Verification items for the finished model (mm, model axes). A direction names the side the tool comes from. Give positions to 0.01 mm unless a question says otherwise; leave off trailing zeros. Loops run counter-clockwise (first coordinate to the right, second up) from the corner with the lowest first, then second, coordinate; pieces in that order, holes last. Notation, with made-up numbers: (30, -17.75) -> (81, -17.75) arc R31 cw to (81, 6.25) -> close; hole circle Ø5 at (19, 3). An arc over 180 degrees is marked (long way). Answer in a Markdown table with one row per item. Add a question column.
Q1. Section check A-A on z = 7.5. Enter the section's corners in (x, y), and give its area (3 significant figures).
Q2. Section check B-B on x = -133. Enter the section's corners in (y, z), and give its area (3 significant figures).
Q3. Gauge pin test, flat ends, axial feed: P1, Ø1.5, axis at y = -55.5, z = 8.5, coming from the +X side; P2, Ø3, axis at x = 122.5, z = 5, coming from the -Y side; P3, Ø3, axis at y = -41.5, z = 1.5, coming from the +X side. Record the tip position at first contact, or that the pin passes through.
Q4. Section check C-C on y = -69. Enter the section's corners in (x, z).
Q5. Set-up check for faces 5 (the face through (-16.557, 26.311, 4.93)), 6 (the face through (120, -25, 5)), 7 (the face through (1, 4, 0)): record each of +Z, -Z, +X, -X, +Y, -Y from which the full face is reachable in a straight line by a thin tool's end or side.
Q6. Material ranges on probe 1 along X at (y, z) = (19, 2); probe 2 along X at (y, z) = (15.5, 5.5); probe 3 along X at (y, z) = (37.5, 3.25), recorded low to high.
Q7. Release check for a two-part mould opening along X. For faces 1 (the face through (142, 50, 5)), 2 (the face through (16.517, 26.689, 4.93)), 3 (the face through (-145.83, -7.04, 4.93)), 4 (the face through (0, 30, 5)) record: pulls with the +X half, pulls with the -X half, needs draft (parallel to the pull), parting line crosses it, or undercut.
```python
from build123d import *

# Parameters (mm, degrees)
BOSS_EXTRUDE1_DEPTH = 10


with BuildPart() as part:
    # Sketch1 → Boss-Extrude1 (new body)
    with BuildSketch(Plane.XY):
        with BuildLine():
            Line((67, 50), (220, 50))
            Line((220, 50), (158.952536164, 7.254105633))
            ThreePointArc((158.952536164, 7.254105633), (145.965681261, -6.810123789), (140, -25))
            Line((140, -25), (99.563224144, -25))
            ThreePointArc((99.563224144, -25), (32.234251016, -51.062124878), (0, -115.663812449))
            ThreePointArc((0, -115.663812449), (-32.234251016, -51.062124878), (-99.563224144, -25))
            Line((-99.563224144, -25), (-140, -25))
            ThreePointArc((-140, -25), (-145.965681261, -6.810123789), (-158.952536164, 7.254105633))
            Line((-158.952536164, 7.254105633), (-220, 50))
            Line((-220, 50), (-67, 50))
            ThreePointArc((-67, 50), (-51.137889855, 20.020793424), (-17.95554779, 13))
            Line((-17.95554779, 13), (-15.117733438, 40))
            Line((-15.117733438, 40), (-12, 27.49545417))
            ThreePointArc((-12, 27.49545417), (0, 30), (12, 27.49545417))
            Line((12, 27.49545417), (15.117733438, 40))
            Line((15.117733438, 40), (17.95554779, 13))
            ThreePointArc((17.95554779, 13), (51.137889855, 20.020793424), (67, 50))
        make_face()
    extrude(amount=BOSS_EXTRUDE1_DEPTH)


solid = part.part
```
Taken from the geometry:
| question | item | result |
|---|---|---|
| 1 | outline | (-220, 50) -> (-158.95, 7.25) arc R45 cw to (-140, -25) -> (-99.56, -25) arc R100 cw to (0, -115.66) arc R100 cw to (99.56, -25) -> (140, -25) arc R45 cw to (158.95, 7.25) -> (220, 50) -> (67, 50) arc R40 cw to (17.96, 13) -> (15.12, 40) -> (12, 27.5) arc R30 ccw to (-12, 27.5) -> (-15.12, 40) -> (-17.96, 13) arc R40 cw to (-67, 50) -> close |
| 1 | area | 26,100 mm² |
| 2 | outline | (-25, 0) -> (50, 0) -> (50, 10) -> (-25, 10) -> close |
| 2 | area | 750 mm² |
| 3 | P1 | stops at x = 28.39 |
| 3 | P2 | stops at y = -25 |
| 3 | P3 | stops at x = 46.88 |
| 4 | outline | (-16.71, 0) -> (16.71, 0) -> (16.71, 10) -> (-16.71, 10) -> close |
| 5 | face 5 | +Z, -Z, +Y |
| 5 | face 6 | +Z, -Z, +X, -Y |
| 5 | face 7 | -Z, +X, -X, +Y, -Y |
| 6 | probe 1 | x = -175.73 to -49.72, -17.32 to 17.32, 49.72 to 175.73 |
| 6 | probe 2 | x = -170.73 to -43.52, -17.69 to 17.69, 43.52 to 170.73 |
| 6 | probe 3 | x = -202.15 to -64.35, -15.38 to -14.49, 14.49 to 15.38, 64.35 to 202.15 |
| 7 | face 1 | needs draft |
| 7 | face 2 | undercut |
| 7 | face 3 | pulls with the -X half |
| 7 | face 4 | undercut |
